from build123d import *

# Parameters (mm, degrees)
F0_W     = 60
F0_H     = 18
F1_DEPTH = 1500
F2_W     = 100
F2_H     = 60
F3_DEPTH = 300
F4_R     = 20
F5_DEPTH = 96


with BuildPart() as f1:
    # F0 (on Right) → F1 (new body)
    with BuildSketch(Plane.YZ):
        with Locations((-39.5727836765, 84.7336053236)):
            Rectangle(F0_W, F0_H)
    extrude(amount=F1_DEPTH)



with BuildPart() as f1b:
    # F0 (on Right) → F1, piece 2 (new body)
    with BuildSketch(Plane.YZ):
        with Locations((80.4272163235, 84.7336053236)):
            Rectangle(F0_W, F0_H)
    extrude(amount=F1_DEPTH)


with BuildPart() as f1c:
    # F0 (on Right) → F1, piece 3 (new body)
    with BuildSketch(Plane.YZ):
        with Locations((200.4272163235, 84.7336053236)):
            Rectangle(F0_W, F0_H)
    extrude(amount=F1_DEPTH)


with BuildPart() as f1d:
    # F0 (on Right) → F1, piece 4 (new body)
    with BuildSketch(Plane.YZ):
        with Locations((-39.5727836765, 6.7336053236)):
            Rectangle(F0_W, F0_H)
    extrude(amount=F1_DEPTH)


with BuildPart() as f1e:
    # F0 (on Right) → F1, piece 5 (new body)
    with BuildSketch(Plane.YZ):
        with Locations((80.4272163235, 6.7336053236)):
            Rectangle(F0_W, F0_H)
    extrude(amount=F1_DEPTH)


with BuildPart() as f1f:
    # F0 (on Right) → F1, piece 6 (new body)
    with BuildSketch(Plane.YZ):
        with Locations((200.4272163235, 6.7336053236)):
            Rectangle(F0_W, F0_H)
    extrude(amount=F1_DEPTH)


with BuildPart() as f1_1:
    add(f1.part)

    add(f1b.part)  # F3 merges F1b

    add(f1c.part)  # F3 merges F1c

    add(f1d.part)  # F3 merges F1d

    add(f1e.part)  # F3 merges F1e

    add(f1f.part)  # F3 merges F1f
    # F2 (on face) → F3 (join)
    with BuildSketch(Plane(origin=(0, 230.4272163235, 0), x_dir=(-1, 0, 0), z_dir=(0, 1, 0))):
        with Locations((-350, 45.7336053236)):
            Rectangle(F2_W, F2_H)
        with Locations((-550, 45.7336053236)):
            Rectangle(F2_W, F2_H)
        with Locations((-750, 45.7336053236)):
            Rectangle(F2_W, F2_H)
        with Locations((-950, 45.7336053236)):
            Rectangle(F2_W, F2_H)
        with Locations((-1150, 45.7336053236)):
            Rectangle(F2_W, F2_H)
    extrude(amount=-F3_DEPTH)

    # F4 (on face) → F5 (cut, through all)
    with BuildSketch(Plane.XY.offset(93.7336053236)):
        with Locations((50, 80.4272163235)):
            Circle(F4_R)
        with Locations((1450, 80.4272163235)):
            Circle(F4_R)
    extrude(amount=-F5_DEPTH, mode=Mode.SUBTRACT)


solid = f1_1.part
Input: part model. Units: mm. Frame: model coordinates. A direction names the side the tool comes from. Give positions to 0.01 mm unless a question says otherwise; leave off trailing zeros. Write each loop counter-clockwise with the first axis right and the second up, starting at its lowest first coordinate (ties: lowest second). Pieces come first, ordered by that corner, then holes. Notation, with made-up numbers: (20.5, 3) -> (59.5, 3) arc R23 cw to (59.5, 33) -> close; hole circle Ø6 at (58, 27.25). An arc over 180 degrees is marked (long way). Use one line per item in the form item = value. Start each with the question number.
1) Section query A-A on z = 58. Return the cut outline in (x, y).
2) Section query C-C on y = 155. Return the cut outline in (x, z), then the cut area to 3 significant figures.
3) Section query D-D on x = 274. Return the cut outline in (y, z), then the cut area to 3 significant figures.
4) Set-up query: faces 3 (the flat face through (148, 80, 15.734)), 4 (the flat face through (1049, 80, 75.734)), 5 (the flat face through (751, 21, 15.734)), 6 (the flat face through (1348, 80, 15.734)). Return all of +Z, -Z, +X, -X, +Y, -Y with unobstructed straight access to the full face (end or side cutting, diameter ignored); none if empty.
5) Draft query along X for faces 1 (the flat face through (351, 141, 15.734)), 2 (the flat face through (900, 83, 45)). Return one class per face: pulls with the +X half, pulls with the -X half, needs draft (parallel to the pull), parting line crosses it, or undercut.
6) Ray query, probe 1 along Y at (x, z) = (50, 83.75); probe 2 along X at (y, z) = (141, 18); probe 3 along Y at (x, z) = (1411, 82.5). Return the intervals inside material, ascending. Write a range as from..to.
7) Section query B-B on x = 1450. Count the separate pieces of the cut face and the enclosed holes in it, then the cut area to 3 significant figures.
8) Pin query (flat end, axial travel): pin 1 (1 mm diameter, centred on y = -23, z = 30.5, fed in from +X); pin 2 (18 mm diameter, centred on x = 562, y = 18.5, fed in from +Z); pin 3 (18 mm diameter, centred on y = 49, z = 50, fed in from -X). Return the tip coordinate at first contact, or that it passes through.
Outcome:
q1.outline = (300, -69.57) -> (400, -69.57) -> (400, 230.43) -> (300, 230.43) -> close; (500, -69.57) -> (600, -69.57) -> (600, 230.43) -> (500, 230.43) -> close; (700, -69.57) -> (800, -69.57) -> (800, 230.43) -> (700, 230.43) -> close; (900, -69.57) -> (1000, -69.57) -> (1000, 230.43) -> (900, 230.43) -> close; (1100, -69.57) -> (1200, -69.57) -> (1200, 230.43) -> (1100, 230.43) -> close
q2.outline = (300, 15.73) -> (400, 15.73) -> (400, 75.73) -> (300, 75.73) -> close; (500, 15.73) -> (600, 15.73) -> (600, 75.73) -> (500, 75.73) -> close; (700, 15.73) -> (800, 15.73) -> (800, 75.73) -> (700, 75.73) -> close; (900, 15.73) -> (1000, 15.73) -> (1000, 75.73) -> (900, 75.73) -> close; (1100, 15.73) -> (1200, 15.73) -> (1200, 75.73) -> (1100, 75.73) -> close
q2.area = 30,000 mm^2
q3.outline = (-69.57, -2.27) -> (-9.57, -2.27) -> (-9.57, 15.73) -> (-69.57, 15.73) -> close; (-69.57, 75.73) -> (-9.57, 75.73) -> (-9.57, 93.73) -> (-69.57, 93.73) -> close; (50.43, -2.27) -> (110.43, -2.27) -> (110.43, 15.73) -> (50.43, 15.73) -> close; (50.43, 75.73) -> (110.43, 75.73) -> (110.43, 93.73) -> (50.43, 93.73) -> close; (170.43, -2.27) -> (230.43, -2.27) -> (230.43, 15.73) -> (170.43, 15.73) -> close; (170.43, 75.73) -> (230.43, 75.73) -> (230.43, 93.73) -> (170.43, 93.73) -> close
q3.area = 6,480 mm^2
q4.face_3 = -X, +Y, -Y
q4.face_4 = +Y, -Y
q4.face_5 = -Z, +X, -X
q4.face_6 = +X, +Y, -Y
q5.face_1 = needs draft
q5.face_2 = undercut
q6.probe_1 = -69.57..-9.57, 50.43..60.43, 100.43..110.43, 170.43..230.43
q6.probe_2 = 300..400, 500..600, 700..800, 900..1000, 1100..1200
q6.probe_3 = -69.57..-9.57, 50.43..110.43, 170.43..230.43
q7.separate_pieces = 8
q7.enclosed_holes = 0
q7.area = 5,040 mm^2
q8.pin_1 = 1200
q8.pin_2 = 75.73
q8.pin_3 = 300
